from build123d import *

# Parameters (mm, degrees)
SKETCH_1_R               = 2.15
EXTRUDE_1_DEPTH          = 40
CUT_EXTRUDE_2_DEPTH      = 58.739891142
CUT_EXTRUDE_2_DEPTH_BACK = 10
SKETCH_2_W               = 10.1
SKETCH_2_H               = 10
SKETCH_4_W               = 40
SKETCH_4_H               = 4
EXTRUDE_2_DEPTH          = 2
CUT_EXTRUDE_3_DEPTH      = 3.5
FILLET_1_R               = 8


with BuildPart() as part:
    # 草图1 → 凸台-拉伸1 (new body)
    with BuildSketch(Plane.XY):
        with BuildLine():
            Line((-20, 1.75), (-22.225540425, 3.975540425))
            ThreePointArc((-22.225540425, 3.975540425), (-23.242576583, 10.851086981), (-26.419060249, 4.669060249))
            Line((-26.419060249, 4.669060249), (-20, -1.75))
            Line((-20, -1.75), (20, -1.75))
            Line((20, -1.75), (20, 1.75))
            Line((20, 1.75), (-20, 1.75))
        make_face()
        with Locations((-23.838120497, 7.25)):
            Circle(SKETCH_1_R, mode=Mode.SUBTRACT)
    extrude(amount=EXTRUDE_1_DEPTH)

    # 草图2 → 切除-拉伸2 (cut, two sides: drawn at the far end of the back side and taken through both)
    with BuildSketch(Plane(origin=(-20.188120497, 0, 0), x_dir=(0, 0, -1), z_dir=(1, 0, 0)).offset(-CUT_EXTRUDE_2_DEPTH_BACK)):
        with Locations((-29.95, 6.75)):
            Rectangle(SKETCH_2_W, SKETCH_2_H)
        with Locations((-10.05, 6.75)):
            Rectangle(SKETCH_2_W, SKETCH_2_H)
    extrude(amount=CUT_EXTRUDE_2_DEPTH + CUT_EXTRUDE_2_DEPTH_BACK, mode=Mode.SUBTRACT)

    # 草图4 → 凸台-拉伸2 (add)
    with BuildSketch(Plane.XZ.offset(1.75)):
        with Locations((0, 2)):
            Rectangle(SKETCH_4_W, SKETCH_4_H)
        with Locations((0, 38)):
            Rectangle(SKETCH_4_W, SKETCH_4_H)
    extrude(amount=EXTRUDE_2_DEPTH)

    # 草图5 → 切除-拉伸3 (cut)
    with BuildSketch(Plane(origin=(0, 1.75, 0), x_dir=(1, 0, 0), z_dir=(0, 1, 0))):
        with BuildLine():
            Line((11.414328277, -30.822898901), (-11.445671723, -30.822898901))
            ThreePointArc((-11.445671723, -30.822898901), (-12.343697335, -31.194873288), (-12.715671723, -32.092898901))
            Line((-12.715671723, -32.092898901), (-12.715671723, -33.362898901))
            ThreePointArc((-12.715671723, -33.362898901), (-12.343697335, -34.260924513), (-11.445671723, -34.632898901))
            Line((-11.445671723, -34.632898901), (11.414328277, -34.632898901))
            ThreePointArc((11.414328277, -34.632898901), (12.31235389, -34.260924513), (12.684328277, -33.362898901))
            Line((12.684328277, -33.362898901), (12.684328277, -32.092898901))
            ThreePointArc((12.684328277, -32.092898901), (12.31235389, -31.194873288), (11.414328277, -30.822898901))
        make_face()
        with BuildLine():
            Line((12.684328277, -7.962898901), (12.684328277, -6.692898901))
            ThreePointArc((12.684328277, -6.692898901), (12.31235389, -5.794873288), (11.414328277, -5.422898901))
            Line((11.414328277, -5.422898901), (-11.445671723, -5.422898901))
            ThreePointArc((-11.445671723, -5.422898901), (-12.343697335, -5.794873288), (-12.715671723, -6.692898901))
            Line((-12.715671723, -6.692898901), (-12.715671723, -7.962898901))
            ThreePointArc((-12.715671723, -7.962898901), (-12.343697335, -8.860924513), (-11.445671723, -9.232898901))
            Line((-11.445671723, -9.232898901), (11.414328277, -9.232898901))
            ThreePointArc((11.414328277, -9.232898901), (12.31235389, -8.860924513), (12.684328277, -7.962898901))
        make_face()
    extrude(amount=-CUT_EXTRUDE_3_DEPTH, mode=Mode.SUBTRACT)

    # 圆角1
    # the kernel refuses this fillet: 8 mm, written as the material it adds along each edge
    with BuildSketch(Plane(origin=(-20, -1.75, 0), x_dir=(-0.707106781186549, 0.7071067811865461, 0), z_dir=(0, 0, 1)), Plane(origin=(-20, -1.75, 36), x_dir=(-0.707106781186549, 0.7071067811865461, 0), z_dir=(0, 0, 1))) as fillet_1_piece_1:
        with BuildLine():
            CenterArc((3.127528064, 8), FILLET_1_R, 235.408772886, 34.591227114)
            Line((-1.414213562, 1.414213562), (0, 0))
            Line((0, 0), (3.127528064, 0))
        make_face()
    extrude(amount=4)
    with BuildSketch(Plane(origin=(-20, 1.75, 0), x_dir=(-0.7071067811865483, 0.7071067811865467, 0), z_dir=(0, 0, 1))) as fillet_1_piece_2:
        with BuildLine():
            CenterArc((3.31547448, -7.998234019), FILLET_1_R, 91.203908923, 43.796091077)
            Line((-2.34137977, -2.34137977), (0, 0))
            Line((0, 0), (3.147389452, 0))
        make_face()
    extrude(amount=5)
    with BuildSketch(Plane(origin=(-20, 1.75, 15.1), x_dir=(1, 0, 0), z_dir=(0, 0, 1))) as fillet_1_piece_3:
        with BuildLine():
            CenterArc((3.311211025, 8), FILLET_1_R, 226.203908923, 43.796091077)
            Line((-2.225540425, 2.225540425), (0, 0))
            Line((0, 0), (3.311211025, 0))
        make_face()
    extrude(amount=9.8)
    with BuildSketch(Plane(origin=(-20, 1.75, 35), x_dir=(1, 0, 0), z_dir=(0, 0, 1))) as fillet_1_piece_4:
        with BuildLine():
            CenterArc((3.311211025, 8), FILLET_1_R, 226.203908923, 43.796091077)
            Line((-2.225540425, 2.225540425), (0, 0))
            Line((0, 0), (3.311211025, 0))
        make_face()
    extrude(amount=5)


solid = part.part
Check sheet for the modelled part. Datum: model origin and axes. Units: mm. A direction names the side the tool comes from. Give positions to 0.01 mm unless a question says otherwise; leave off trailing zeros. Write each loop counter-clockwise with the first axis right and the second up, starting at its lowest first coordinate (ties: lowest second). Pieces come first, ordered by that corner, then holes. Notation, with made-up numbers: (-37.5, -1) -> (-8.5, -1) arc R28 ccw to (-8.5, 19) -> close; hole circle Ø6 at (-36.75, 42). An arc over 180 degrees is marked (long way). One line per item, written item: value. Start each with the question number.
Item 1: Section check D-D on y = -3. Record the cut outline in (x, z), then the cut area to 3 significant figures.
Item 2: Section check C-C on z = 37. Record the cut outline in (x, y), then the cut area to 3 significant figures.
Item 3: Section check A-A on x = -6.5. Record the cut outline in (y, z).
Item 4: Section check B-B on y = 7.25. Record the cut outline in (x, z).
Item 5: Gauge pin test, flat ends, axial feed: pin 1 (10 mm diameter, centred on x = -4.5, z = 17.5, fed in from +Y); pin 2 (2 mm diameter, centred on x = -5, z = 14.5, fed in from -Y); pin 3 (0.6 mm diameter, centred on y = -0.5, z = 7.5, fed in from -X). Record the tip position at first contact, or that the pin passes through.
Item 6: Material ranges on probe 1 along Z at (x, y) = (3, 1.5); probe 2 along Z at (x, y) = (-21, 6); probe 3 along Z at (x, y) = (17.5, -3), recorded low to high. Write a range as from..to.
Item 7: Draft check along X on faces 3 (the flat face through (-12.716, 0, 33)), 4 (the flat face through (-24.5, 5, 24.9)), 5 (the cylindrical face through (-20.77, -1.51, 1.97)). Enter one of: +X half, -X half, draft (parallel to the pull), parting line (faces both ways), or undercut.
Item 8: Tool access check on faces 1 (the flat face through (0, -3.75, 2)), 2 (the flat face through (-12.716, 0, 7)). Record the directions out of +Z, -Z, +X, -X, +Y, -Y that give a thin tool (end or side, any length) a straight path to the whole face; none if there is none.
Results list:
1. outline: (-20.18, 0) -> (20, 0) -> (20, 4) -> (-20.18, 4) -> close; (-20.18, 36) -> (20, 36) -> (20, 40) -> (-20.18, 40) -> close
1. area: 321 mm²
2. outline: (-26.42, 4.67) -> (-22.21, 0.46) arc R8 cw to (-20, -3.75) -> (20, -3.75) -> (20, 1.75) -> (-16.69, 1.75) arc R8 cw to (-22.23, 3.98) arc R3.65 ccw (long way) to start; hole circle Ø4.3 at (-23.84, 7.25)
2. area: 263 mm²
3. outline: (-3.75, 0) -> (1.75, 0) -> (1.75, 5.42) -> (-1.75, 5.42) -> (-1.75, 4) -> (-3.75, 4) -> close; (-3.75, 36) -> (-1.75, 36) -> (-1.75, 34.63) -> (1.75, 34.63) -> (1.75, 40) -> (-3.75, 40) -> close; (-1.75, 9.23) -> (1.75, 9.23) -> (1.75, 30.82) -> (-1.75, 30.82) -> close
4. outline: (-27.49, 0) -> (-25.99, 0) -> (-25.99, 5) -> (-27.49, 5) -> close; (-27.49, 15.1) -> (-25.99, 15.1) -> (-25.99, 24.9) -> (-27.49, 24.9) -> close; (-27.49, 35) -> (-25.99, 35) -> (-25.99, 40) -> (-27.49, 40) -> close; (-21.69, 0) -> (-20.19, 0) -> (-20.19, 5) -> (-21.69, 5) -> close; (-21.69, 15.1) -> (-20.19, 15.1) -> (-20.19, 24.9) -> (-21.69, 24.9) -> close; (-21.69, 35) -> (-20.19, 35) -> (-20.19, 40) -> (-21.69, 40) -> close
5. pin 1: y = 1.75
5. pin 2: y = -1.75
5. pin 3: x = -21.55
6. probe 1: 0..5.42, 9.23..30.82, 34.63..40
6. probe 2: 0..5, 15.1..24.9, 35..40
6. probe 3: 0..4, 36..40
7. face 3: undercut
7. face 4: draft
7. face 5: -X half
8. face 1: +Z, -Z, +X, -X, -Y
8. face 2: +Y, -Y
